Autodesk Inventor part; units mm, degrees
ref_plane "YZ Plane" through (0, 0, 0) normal (1, 0, 0) x (0, 1, 0)
ref_plane "XZ Plane" through (0, 0, 0) normal (0, 1, 0) x (-1, 0, 0)
ref_plane "XY Plane" through (0, 0, 0) normal (0, 0, 1) x (1, 0, 0)
sketch "Sketch1" plane through (0, 0, 0) normal (0, 0, 1) x (1, 0, 0)
  line L0 (-39, 50) -> (6, 50)
  line L1 (6, 50) -> (6, 44)
  line L2 (6, 44) -> (-39, 44)
  line L3 (-39, 44) -> (-39, 50)
  line L4 (0, 44) -> (6, 44)
  line L5 (6, 44) -> (6, 0)
  line L6 (6, 0) -> (0, 0)
  line L7 (0, 0) -> (0, 44)
  dimension "d1" = 6
  dimension "d2" = 45
  dimension "d3" = 6
  dimension "d17" = 50
extrude "Extrusion1" add sketch "Sketch1" along normal blind 3
fillet "Fillet1" radius 15 1 edges at (0, 44, 1.5)
sketch "Sketch2" plane through (0, 0, 3) normal (0, 0, 1) x (1, 0, 0)
  line L0 (6, 50) -> (-39, 50)
  line L1 (6, 0) -> (6, 50)
  point P0 (0, 0)
  point P1 (0, 44)
  dimension "d8" = 6
  dimension "d9" = 6
hole "Hole1" at (0, 44, 3) direction (0, 0, -1) diameter 6 end through all
equation "\"d3\" = d1"
properties part number "Selection_Selector 1" material "Nylon 6/6"
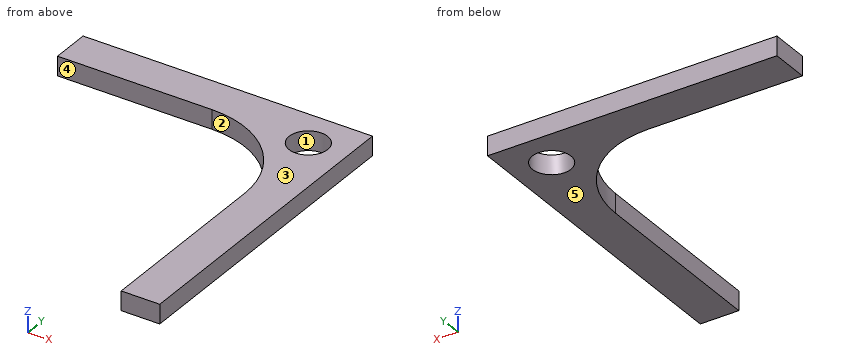
Model file for the job. Use its own axes, mm. Face numbers are marked on the shaded views. A direction names the side the tool comes from. Coordinates: 2 decimals unless noted, no trailing zeros. Loops run counter-clockwise (first coordinate to the right, second up) from the corner with the lowest first, then second, coordinate; pieces in that order, holes last. Notation, with made-up numbers: (-36.5, 7) - (4.5, 7) arc R6 ccw to (4.5, 16) - close; hole circle Ø6 at (82.5, 11). An arc over 180 degrees is marked (long way). Write item = value, one per line. Start each with the question number.
Item 1: Saw through at B-B, the plane y = 43. List the corners of the cut face in (x, z), then the cut area to 3 significant figures.
Item 2: Saw through at A-A, the plane z = 1.2. List the corners of the cut face in (x, y).
Item 3: Wall check: probe 1 along Y at (x, z) = (-19.5, 2.5); probe 2 along X at (y, z) = (42, 1.1); probe 3 along X at (y, z) = (46.5, 1.7). Give the ranges that are in metal, low to high. Write a range as [from, to].
Item 4: Drop flat-ended pins along their axis: pin 1 Ø1.5 at (y, z) = (18.5, 2) entering from -X; pin 2 Ø8 at (x, y) = (-0.5, 21) entering from +Z. Give the stop position or say it passes through.
Item 5: 3-axis set-ups, long thin cutter, end or side, ignore diameter. For the marked faces 4 and 5: which of +Z, -Z, +X, -X, +Y, -Y reach the whole face in a straight line?
Item 6: Pull direction Y, two halves, no side cores. Call the marked faces 1, 2 and 3: +Y half, -Y half, draft (parallel to the pull), parting line (faces both ways), or undercut.
Item 7: Saw through at D-D, the plane y = 17. List the corners of the cut face in (x, z).
Item 8: Saw through at C-C, the plane x = -1. List the corners of the cut face in (y, z), then the cut area to 3 significant figures.
Answers:
q1.outline = (-9.61, 0) - (-2.83, 0) - (-2.83, 3) - (-9.61, 3) - close; (2.83, 0) - (6, 0) - (6, 3) - (2.83, 3) - close
q1.area = 29.9 mm2
q2.outline = (-39, 44) - (-15, 44) arc R15 cw to (0, 29) - (0, 0) - (6, 0) - (6, 50) - (-39, 50) - close; hole circle Ø6 at (0, 44)
q3.probe_1 = [44, 50]
q3.probe_2 = [-7.52, -2.24], [2.24, 6]
q3.probe_3 = [-39, -1.66], [1.66, 6]
q4.pin_1 = 0
q4.pin_2 = 3
q5.face_4 = +Z, -Z, -X, -Y
q5.face_5 = -Z, +X, -X, +Y, -Y
q6.face_1 = undercut
q6.face_2 = -Y half
q6.face_3 = draft
q7.outline = (0, 0) - (6, 0) - (6, 3) - (0, 3) - close
q8.outline = (34.39, 0) - (41.17, 0) - (41.17, 3) - (34.39, 3) - close; (46.83, 0) - (50, 0) - (50, 3) - (46.83, 3) - close
q8.area = 29.9 mm2
